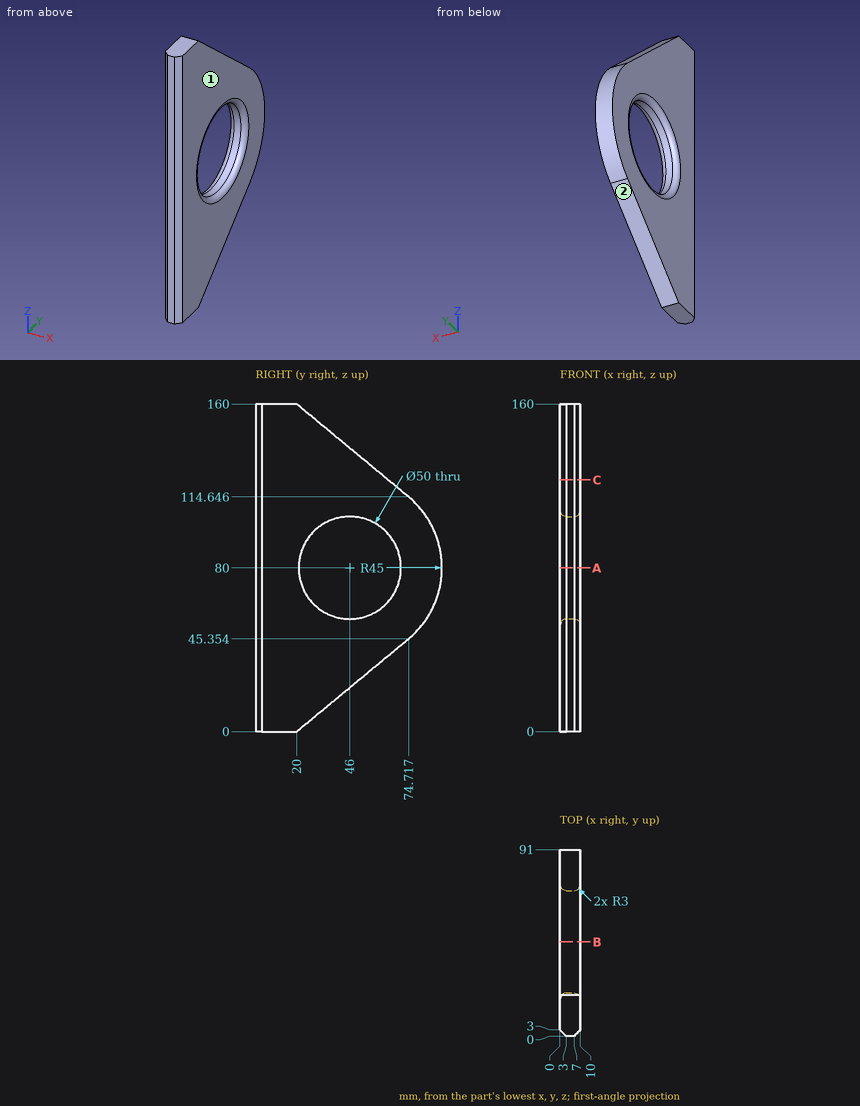
Can you work these out from the drawing? Everything is in mm from the part's minimum corner. Give positions to 0.01 mm unless a question says otherwise; leave off trailing zeros. Loops run counter-clockwise (first coordinate to the right, second up) from the corner with the lowest first, then second, coordinate; pieces in that order, holes last. Notation, with made-up numbers: (-20.5, -23.75) -> (-14.5, -23.75) arc R14 ccw to (-14.5, -4.75) -> close; hole circle Ø2 at (9, 1.25). An arc over 180 degrees is marked (long way). Put each result on its own line as item: value.
(1) Imagine slicing it at A-A on z = 80. Write out the boundary of the cut face in (x, y).
Computed:
outline: (0, 3) -> (3, 0) -> (7, 0) -> (10, 3) -> (10, 18) arc R3 ccw to (7, 21) -> (3, 21) arc R3 ccw to (0, 18) -> close; (0, 74) arc R3 ccw to (3, 71) -> (7, 71) arc R3 ccw to (10, 74) -> (10, 91) -> (0, 91) -> close
(2) Thinking about a two-plate mould opening in Y: for the marked faces 1 and 2, which applies, pulls with the +Y half, pulls with the -Y half, needs draft (parallel to the pull), parting line crosses it, or undercut?
Computed:
face 1: needs draft
face 2: pulls with the +Y half
(3) Imagine slicing it at B-B on y = 46. Write out the boundary of the cut face in (x, z), plus the area to 3 significant figures.
Computed:
outline: (0, 21.55) -> (10, 21.55) -> (10, 52) arc R3 ccw to (7, 55) -> (3, 55) arc R3 ccw to (0, 52) -> close; (0, 108) arc R3 ccw to (3, 105) -> (7, 105) arc R3 ccw to (10, 108) -> (10, 138.45) -> (0, 138.45) -> close
area: 661 mm^2
(4) Imagine slicing it at C-C on z = 123. Write out the boundary of the cut face in (x, y).
Computed:
outline: (0, 3) -> (3, 0) -> (7, 0) -> (10, 3) -> (10, 64.64) -> (0, 64.64) -> close
(5) I'm going to push flat-ended pins straight in: pin 1 Ø1.5 at (x, y) = (7.5, 56.5) entering from -Z; pin 2 Ø3 at (x, y) = (1.5, 72.5) entering from +Z. Where does each tip first touch, or does it pass through?
Computed:
pin 1: z = 29.63
pin 2: z = 117.73
(6) Please list where these lines run through material, in increasing order: probe 1 along Y at (x, z) = (5.95, 80); probe 2 along Y at (x, z) = (3, 94.5) (1 decimal); probe 3 along Y at (x, z) = (3, 41) (1 decimal). Write a range as [from, to].
Computed:
probe 1: [0, 21], [71, 91]
probe 2: [0, 25.6], [66.4, 88.6]
probe 3: [0, 69.5]
